Design review of the part built by this model. Coordinates are the model's own, in mm. A direction names the side the tool comes from. Coordinates: 2 decimals unless noted, no trailing zeros. Loops run counter-clockwise (first coordinate to the right, second up) from the corner with the lowest first, then second, coordinate; pieces in that order, holes last. Notation, with made-up numbers: (9.5, 34.5) - (65.5, 34.5) arc R30 ccw to (65.5, 68.5) - close; hole circle Ø4 at (89, 58). An arc over 180 degrees is marked (long way). Answer in a Markdown table with one row per item. Add a question column.
(1) For faces 1 (the face through (-27, -7, -35)), 2 (the face through (33, -2, -20)), 3 (the face through (38.14, 8.6, -0.53)), list the 3-axis set-ups (+Z, -Z, +X, -X, +Y, -Y) from which the entire face can be reached by the end or side of a thin tool; tool diameter is ignored.
(2) Clearance check with flat-ended pins moving along their axes: pin 1 (1.2 mm diameter, centred on y = -7.5, z = -32.5, fed in from -X); pin 2 (1.2 mm diameter, centred on x = -26, z = -32.5, fed in from -Y); pin 3 (1.8 mm diameter, centred on x = 33.5, y = -2.5, fed in from -Z). State where each tip first meets the part, or that it passes through.
(3) To check wall thickness, follow L1, parallel to Y at x = 33, z = -33.75; L2, parallel to X at y = -7, z = -32.5; L3, parallel to X at y = 7.5, z = -7. State the ranges of each line that lie inside material, in increasing order. Write a range as [from, to].
(4) The part is to be moulded in two halves that separate along Y. For faces 4 (the face through (-27, -4.5, -33)), 5 (the face through (-38.14, 8.6, 0.53)), 6 (the face through (34.75, -2.42, -29.63)), 7 (the face through (39, 0, 1)), say which applies: released by +Y, released by -Y, zero draft, split by the parting line, or undercut.
(5) We need section A-A, the plane x = 33. Write out the cut boundary in (y, z), plus the area to 3 significant figures.
from build123d import *

# Parameters (mm, degrees)
SKETCH1_W           = 78
SKETCH1_H           = 78
BOSS_EXTRUDE1_DEPTH = 9.5
SKETCH2_R           = 1.75
CUT_EXTRUDE1_DEPTH  = 19
SKETCH3_W           = 6
SKETCH3_H           = 4
CUT_EXTRUDE2_DEPTH  = 5
FILLET2_R           = 1
FILLET3_R           = 3
FILLET4_R           = 1


with BuildPart() as part:
    # Sketch1 → Boss-Extrude1 (new, symmetric)
    with BuildSketch(Plane(origin=(0, 0, 0), x_dir=(1, 0, 0), z_dir=(0, 1, 0))):
        Rectangle(SKETCH1_W, SKETCH1_H)
    extrude(amount=BOSS_EXTRUDE1_DEPTH, both=True)

    # Sketch2 → Cut-Extrude1 (cut)
    with BuildSketch(Plane(origin=(0, 0, -39), x_dir=(-1, 0, 0), z_dir=(0, 0, -1))):
        with Locations((-33, -2.5)):
            Circle(SKETCH2_R)
    extrude(amount=-CUT_EXTRUDE1_DEPTH, mode=Mode.SUBTRACT)

    # Sketch3 → Cut-Extrude2 (cut)
    with BuildSketch(Plane.XZ.offset(9.5)):
        with Locations((-27.1, -33)):
            Rectangle(SKETCH3_W, SKETCH3_H)
    extrude(amount=-CUT_EXTRUDE2_DEPTH, mode=Mode.SUBTRACT)

    # Fillet2
    fillet2_edges = [part.edges().sort_by_distance(p)[0] for p in [
        (0, -9.5, -39),
        (-39, 0, -39),
        (39, 0, -39),
        (0, 9.5, -39),
    ]]
    fillet(fillet2_edges, radius=FILLET2_R)

    # Fillet3
    # the kernel refuses this fillet: 3 mm, written as the material it takes off along each edge
    with BuildSketch(Plane(origin=(36, 6.5, -39), x_dir=(0, 1, 0), z_dir=(-1, 0, 0))) as fillet3_piece_1:
        with BuildLine():
            CenterArc((2, -1), 1, 0, 90)
            Line((3, -1), (3, 0))
            Line((3, 0), (2, 0))
        make_face()
    revolve(axis=Axis((36, 6.5, -39), (0, 0, -1)), revolution_arc=90, mode=Mode.SUBTRACT)
    with BuildSketch(Plane(origin=(36, -6.5, -39), x_dir=(1, 0, 0), z_dir=(0, 1, 0))) as fillet3_piece_2:
        with BuildLine():
            CenterArc((2, -1), 1, 0, 90)
            Line((3, -1), (3, 0))
            Line((3, 0), (2, 0))
        make_face()
    revolve(axis=Axis((36, -6.5, -39), (0, 0, -1)), revolution_arc=90, mode=Mode.SUBTRACT)
    with BuildSketch(Plane(origin=(-36, 6.5, -39), x_dir=(-1, 0, 0), z_dir=(0, -1, 0))) as fillet3_piece_3:
        with BuildLine():
            CenterArc((2, -1), 1, 0, 90)
            Line((3, -1), (3, 0))
            Line((3, 0), (2, 0))
        make_face()
    revolve(axis=Axis((-36, 6.5, -39), (0, 0, -1)), revolution_arc=90, mode=Mode.SUBTRACT)
    with BuildSketch(Plane(origin=(-36, -6.5, -39), x_dir=(0, -1, 0), z_dir=(1, 0, 0))) as fillet3_piece_4:
        with BuildLine():
            CenterArc((2, -1), 1, 0, 90)
            Line((3, -1), (3, 0))
            Line((3, 0), (2, 0))
        make_face()
    revolve(axis=Axis((-36, -6.5, -39), (0, 0, -1)), revolution_arc=90, mode=Mode.SUBTRACT)
    with BuildSketch(Plane(origin=(-39, -9.5, 46.5), x_dir=(1, 0, 0), z_dir=(0, 0, -1)), Plane(origin=(-39, 9.5, 46.5), x_dir=(0, -1, 0), z_dir=(0, 0, -1)), Plane(origin=(39, 9.5, -39), x_dir=(0, -1, 0), z_dir=(0, 0, 1)), Plane(origin=(39, -9.5, -39), x_dir=(-1, 0, 0), z_dir=(0, 0, 1))) as fillet3_piece_5:
        with BuildLine():
            CenterArc((FILLET3_R, -FILLET3_R), FILLET3_R, 90, 90)
            Line((0, -FILLET3_R), (0, 0))
            Line((0, 0), (FILLET3_R, 0))
        make_face()
    extrude(amount=85.5, mode=Mode.SUBTRACT)

    # Fillet4
    fillet4_edges = [part.edges().sort_by_distance(p)[0] for p in [
        (0, 9.5, 39),
        (0, -9.5, 39),
        (39, 0, 39),
        (-39, 0, 39),
        (38.121320344, -8.621320344, 39),
        (38.121320344, 8.621320344, 39),
        (-38.121320344, -8.621320344, 39),
        (-38.121320344, 8.621320344, 39),
    ]]
    fillet(fillet4_edges, radius=FILLET4_R)


solid = part.part
Responses:
| question | item | result |
|---|---|---|
| 1 | face 1 | -Y |
| 1 | face 2 | -Z |
| 1 | face 3 | +Z, -Z, +X, +Y |
| 2 | pin 1 | stops at x = -38.97 |
| 2 | pin 2 | stops at y = -4.5 |
| 2 | pin 3 | stops at z = -20 |
| 3 | L1 | y = [-9.5, -4.25], [-0.75, 9.5] |
| 3 | L2 | x = [-38.96, -30.1], [-24.1, 38.96] |
| 3 | L3 | x = [-38.83, 38.83] |
| 4 | face 4 | released by -Y |
| 4 | face 5 | released by +Y |
| 4 | face 6 | undercut |
| 4 | face 7 | zero draft |
| 5 | outline | (-9.5, -38) arc R1 ccw to (-8.5, -39) - (-4.25, -39) - (-4.25, -20) - (-0.75, -20) - (-0.75, -39) - (8.5, -39) arc R1 ccw to (9.5, -38) - (9.5, 38) arc R1 ccw to (8.5, 39) - (-8.5, 39) arc R1 ccw to (-9.5, 38) - close |
| 5 | area | 1,410 mm2 |
